For this review, take the finished solid that the model builds, in its own axes (mm). A direction names the side the tool comes from. Give positions to 0.01 mm unless a question says otherwise; leave off trailing zeros. Write each loop counter-clockwise with the first axis right and the second up, starting at its lowest first coordinate (ties: lowest second). Pieces come first, ordered by that corner, then holes. Notation, with made-up numbers: (88.5, -27.5) -> (134.5, -27.5) arc R22 ccw to (134.5, -7.5) -> close; hole circle Ø9 at (80, 73). An arc over 180 degrees is marked (long way). Return JSON: item names as keys, results as strings.
from build123d import *

# Parameters (mm, degrees)
SKETCH_1_W          = 200
SKETCH_1_H          = 200
EXTRUDE_1_DEPTH     = 3
SKETCH_2_W          = 2.5
SKETCH_2_H          = 200
EXTRUDE_2_DEPTH     = 20
CUT_EXTRUDE_2_DEPTH = 217.696654335
CUT_EXTRUDE_3_DEPTH = 10


with BuildPart() as part:
    # 草图1 → 凸台-拉伸1 (new body)
    with BuildSketch(Plane(origin=(0, 0, 0), x_dir=(1, 0, 0), z_dir=(0, 1, 0))):
        Rectangle(SKETCH_1_W, SKETCH_1_H)
    extrude(amount=EXTRUDE_1_DEPTH)

    # 草图2 → 凸台-拉伸2 (add)
    with BuildSketch(Plane.XZ):
        with Locations((-66.45, 0)):
            Rectangle(SKETCH_2_W, SKETCH_2_H)
        with Locations((-89.95, 0)):
            Rectangle(SKETCH_2_W, SKETCH_2_H)
    extrude_2 = extrude(amount=EXTRUDE_2_DEPTH)

    # 镜向1: 凸台-拉伸2 across plane
    add(extrude_2.mirror(Plane(origin=(0, 0, 0), x_dir=(0, 0, 1), z_dir=(1, 0, 0))))

    # 草图5 → 切除-拉伸2 (cut, through all)
    with BuildSketch(Plane(origin=(91.2, 0, 0), x_dir=(0, 0, -1), z_dir=(1, 0, 0))):
        with BuildLine():
            Line((-70, -8.25), (70, -8.25))
            ThreePointArc((70, -8.25), (71.75, -10), (70, -11.75))
            Line((70, -11.75), (-70, -11.75))
            ThreePointArc((-70, -11.75), (-71.75, -10), (-70, -8.25))
        make_face()
    extrude(amount=-CUT_EXTRUDE_2_DEPTH, mode=Mode.SUBTRACT)

    # 草图4 → 切除-拉伸3 (cut)
    with BuildSketch(Plane(origin=(0, 3, 0), x_dir=(1, 0, 0), z_dir=(0, 1, 0))):
        Polygon((15.5, -25.5), (15.5, -40.5), (-0.5, -40.5), (-0.5, -25.5), (-25.5, -25.5), (-25.5, 25.5), (25.5, 25.5), (25.5, -25.5), align=None)
    extrude(amount=-CUT_EXTRUDE_3_DEPTH, mode=Mode.SUBTRACT)


solid = part.part
1. For pin 1 (1 mm diameter, centred on x = -69, z = 57, fed in from -Y); pin 2 (10 mm diameter, centred on y = -11, z = 34.5, fed in from +X), all flat-tipped, find the tip position at first contact; note any pin that passes through.
Results found:
{"pin 1": "stops at y = 0", "pin 2": "stops at x = 91.2"}
2. Add section C-C, the plane z = 78. State the section outline as (x, y) points, plus the area to 3 significant figures.
Results found:
{"outline": "(-100, 0) -> (-91.2, 0) -> (-91.2, -20) -> (-88.7, -20) -> (-88.7, 0) -> (-67.7, 0) -> (-67.7, -20) -> (-65.2, -20) -> (-65.2, 0) -> (65.2, 0) -> (65.2, -20) -> (67.7, -20) -> (67.7, 0) -> (88.7, 0) -> (88.7, -20) -> (91.2, -20) -> (91.2, 0) -> (100, 0) -> (100, 3) -> (-100, 3) -> close", "area": "800 mm²"}
3. Add section D-D, the plane z = -19.5. Count the separate pieces of the cut face and the enclosed holes in it, plus the area to 3 significant figures.
Results found:
{"separate pieces": "6", "enclosed holes": "0", "area": "612 mm²"}
4. Add section A-A, the plane x = -6. State the section outline as (y, z) points.
Results found:
{"outline": "(0, -100) -> (3, -100) -> (3, -25.5) -> (0, -25.5) -> close; (0, 25.5) -> (3, 25.5) -> (3, 100) -> (0, 100) -> close"}
5. For faces 1 (the flat face through (91.2, -8, -1)), 2 (the flat face through (-88.7, -8, -1)), 3 (the flat face through (-1, 3, -46)), 4 (the flat face through (-96, 0, -1)), list the 3-axis set-ups (+Z, -Z, +X, -X, +Y, -Y) from which the entire face can be reached by the end or side of a thin tool; tool diameter is ignored.
Results found:
{"face 1": "+Z, -Z, +X, -Y", "face 2": "+Z, -Z, -Y", "face 3": "+Z, -Z, +X, -X, +Y", "face 4": "+Z, -Z, -X, -Y"}
6. The part is to be moulded in two halves that separate along X. For faces 5 (the flat face through (-78, 0, -1)), 6 (the flat face through (88.7, -8, -1)), 7 (the flat face through (-15, 1, 100)), 8 (the flat face through (-91.2, -8, -1)), say which applies: +X half, -X half, draft (parallel to the pull), parting line (faces both ways), or undercut.
Results found:
{"face 5": "undercut", "face 6": "undercut", "face 7": "draft", "face 8": "-X half"}
7. To check wall thickness, follow probe 1 along X at (y, z) = (-3.25, 77); probe 2 along X at (y, z) = (2.25, -4); probe 3 along Y at (x, z) = (-8, -81). State the ranges of each line that lie inside material, in increasing order.
Results found:
{"probe 1": "x = -91.2 to -88.7, -67.7 to -65.2, 65.2 to 67.7, 88.7 to 91.2", "probe 2": "x = -100 to -25.5, 25.5 to 100", "probe 3": "y = 0 to 3"}
8. Add section B-B, the plane y = -2.75. State the section outline as (x, z) points.
Results found:
{"outline": "(-91.2, -100) -> (-88.7, -100) -> (-88.7, 100) -> (-91.2, 100) -> close; (-67.7, -100) -> (-65.2, -100) -> (-65.2, 100) -> (-67.7, 100) -> close; (65.2, -100) -> (67.7, -100) -> (67.7, 100) -> (65.2, 100) -> close; (88.7, -100) -> (91.2, -100) -> (91.2, 100) -> (88.7, 100) -> close"}
